Source: CAD feature listing. Evaluate the final solid. Frame: model axes, mm. Face numbers are marked on the shaded views. A direction names the side the tool comes from. Give positions to 0.01 mm unless a question says otherwise; leave off trailing zeros. Order: outer loops, then holes, each group sorted by start corner. A loop starts at its lowest first (then second) coordinate and runs counter-clockwise, first axis right, second up. Notation, with made-up numbers: M 12,-11.5 L 66,-11.5 A28 cw 66,17.5 Z; hole C 84.5,-35.75 d5. An arc over 180 degrees is marked long. Answer as a JSON object with one key per item and string values. Group by question number.
1. Pin query (flat end, axial travel): P1, Ø5, axis at y = -12, z = 7, coming from the -X side; P2, Ø1.6, axis at x = 0.5, z = 9, coming from the -Y side; P3, Ø0.7, axis at x = 0.5, y = -14, coming from the -Z side; P4, Ø1.8, axis at x = -0.5, z = -1, coming from the +Y side. Return the tip coordinate at first contact, or that it passes through.
2. Section query B-B (x = 1.35). Output: boundary loops of the cut face in (y, z).
3. Section query C-C (z = 1.5). Output: boundary loops of the cut face in (x, y).
4. Section query D-D (y = -17.25). Output: boundary loops of the cut face in (x, z), plus the area to 3 significant figures.
5. Material intervals for L1, parallel to Z at x = 0.1, y = -1.5; L2, parallel to Z at x = -1.2, y = -7.5; L3, parallel to Y at x = 0.15, z = -1.75, sorted ascending. Write a range as [from, to].
6. Section query A-A (y = -2.5). Output: boundary loops of the cut face in (x, z).
7. Pull-direction query (Z, two-part tool) for the marked faces 4, 5, 6 and 7; classes: +Z half, -Z half, draft (parallel to the pull), parting line (faces both ways), or undercut.
8. Set-up query: the marked faces 1, 2 and 3. Return all of +Z, -Z, +X, -X, +Y, -Y with unobstructed straight access to the full face (end or side cutting, diameter ignored); none if empty.
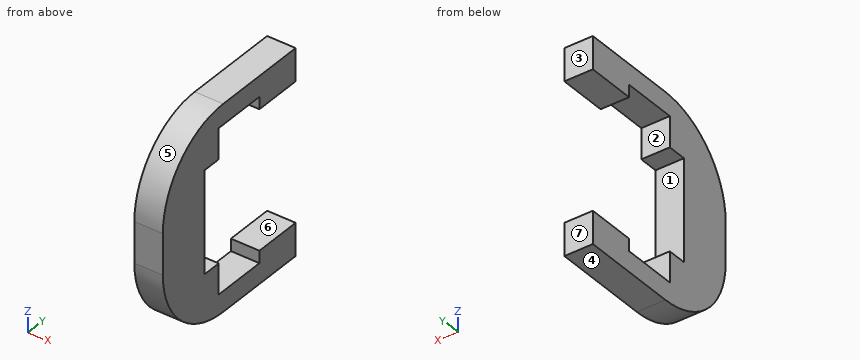
from build123d import *

# Parameters (mm, degrees)
F0_W     = 3.5
F0_H     = 25
F1_DEPTH = 22
F3_DEPTH = 25
F4_R     = 10


with BuildPart() as f1:
    # F0 (on Front) → F1 (new body)
    with BuildSketch(Plane.XZ):
        Rectangle(F0_W, F0_H)
    extrude(amount=F1_DEPTH)

    # F2 (on face) → F3 (cut)
    with BuildSketch(Plane(origin=(-1.75, 0, 0), x_dir=(0, -1, 0), z_dir=(-1, 0, 0))):
        Polygon((0, 8.5), (0, -8.5), (6, -8.5), (6, -10), (12.75, -10), (12.75, -6.25), (15.1, -6.25), (15.1, 6.25), (12.75, 6.25), (12.75, 10), (6, 10), (6, 8.5), align=None)
    extrude(amount=-F3_DEPTH, mode=Mode.SUBTRACT)

    # F4
    f4_edges = [f1.edges().sort_by_distance(p)[0] for p in [
        (0, -22, 12.5),
        (0, -22, -12.5),
    ]]
    fillet(f4_edges, radius=F4_R)


solid = f1.part
Answer sheet:
{
 "1": {"P1": "x = -1.75", "P2": "y = -20.22", "P3": "z = -12.36", "P4": "y = -15.1"},
 "2": {"outline": "M -22,-2.5 A10 ccw -12,-12.5 L 0,-12.5 L 0,-8.5 L -6,-8.5 L -6,-10 L -12.75,-10 L -12.75,-6.25 L -15.1,-6.25 L -15.1,6.25 L -12.75,6.25 L -12.75,10 L -6,10 L -6,8.5 L 0,8.5 L 0,12.5 L -12,12.5 A10 ccw -22,2.5 Z"},
 "3": {"outline": "M -1.75,-22 L 1.75,-22 L 1.75,-15.1 L -1.75,-15.1 Z"},
 "4": {"outline": "M -1.75,-11.01 L 1.75,-11.01 L 1.75,11.01 L -1.75,11.01 Z", "area": "77.1 mm^2"},
 "5": {"L1": "[-12.5, -8.5], [8.5, 12.5]", "L2": "[-12.5, -10], [10, 12.5]", "L3": "[-22, -15.1]"},
 "6": {"outline": "M -1.75,-12.5 L 1.75,-12.5 L 1.75,-8.5 L -1.75,-8.5 Z; M -1.75,8.5 L 1.75,8.5 L 1.75,12.5 L -1.75,12.5 Z"},
 "7": {"face 4": "-Z half", "face 5": "+Z half", "face 6": "undercut", "face 7": "draft"},
 "8": {"face 1": "+X, -X, +Y", "face 2": "+X, -X", "face 3": "+Z, -Z, +X, -X, +Y"}
}
